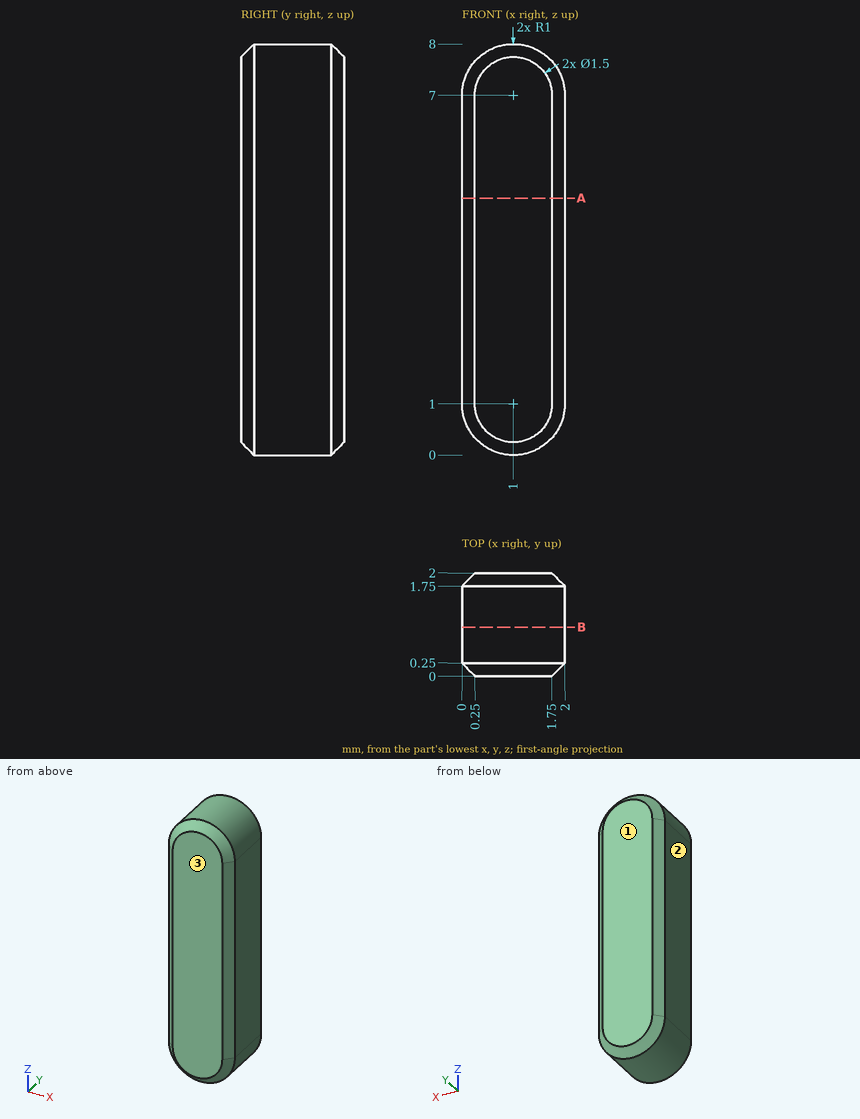
Check sheet for the drawn part. Datum: minimum x, y, z corner. Units: mm. Give positions to 0.01 mm unless a question says otherwise; leave off trailing zeros. Loops run counter-clockwise (first coordinate to the right, second up) from the corner with the lowest first, then second, coordinate; pieces in that order, holes last.
1) Sectioned sample at B-B, the plane y = 0.95. Enter the section's corners in (x, z).
2) Draft check along Y on the marked faces 1, 2 and 3. Enter one of: pulls with the +Y half, pulls with the -Y half, needs draft (parallel to the pull), parting line crosses it, or undercut.
3) Thickness scan on line 1 along Z through (x, y) = (0.9, 1.35); line 2 along X through (y, z) = (0.75, 7.75); line 3 along X through (y, z) = (0.1, 6.5). Record the ranges inside material, lowest first.
4) Sectioned sample at A-A, the plane z = 5. Enter the section's corners in (x, y), then the cut area to 4 significant figures.
Answers:
1. outline: (0, 1) arc R1 ccw to (2, 1) - (2, 7) arc R1 ccw to (0, 7) - close
2. face 1: pulls with the +Y half
2. face 2: needs draft
2. face 3: pulls with the -Y half
3. line 1: z = 0.01 to 7.99
3. line 2: x = 0.34 to 1.66
3. line 3: x = 0.15 to 1.85
4. outline: (0, 0.25) - (0.25, 0) - (1.75, 0) - (2, 0.25) - (2, 1.75) - (1.75, 2) - (0.25, 2) - (0, 1.75) - close
4. area: 3.875 mm2
